Can you work these out from the model? Positions are in its coordinate system, mm. Give positions to 0.01 mm unless a question says otherwise; leave off trailing zeros. Order: outer loops, then holes, each group sorted by start corner. A loop starts at its lowest first (then second) coordinate and runs counter-clockwise, first axis right, second up. Notation, with made-up numbers: (5, 3.25) - (19, 3.25) arc R23 cw to (19, 18.25) - close; hole circle Ø10 at (19, 24.25). An arc over 180 degrees is marked (long way). Return JSON: item names as keys, results as strings.
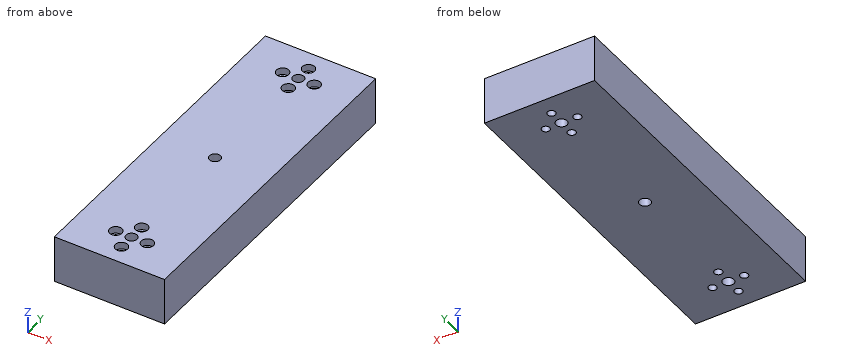
```python
from build123d import *

# Parameters (mm, degrees)
SKETCH1_W                                        = 300
SKETCH1_H                                        = 100
SKETCH1_R                                        = 5
BOSS_EXTRUDE1_DEPTH                              = 42.8
CBORE_FOR_1_4_SOCKET_HEAD_CAP_SCREW1_D           = 7.1374
CBORE_FOR_1_4_SOCKET_HEAD_CAP_SCREW1_CBORE_D     = 11.1125
CBORE_FOR_1_4_SOCKET_HEAD_CAP_SCREW1_CBORE_DEPTH = 6.35


with BuildPart() as part:
    # Sketch1 → Boss-Extrude1 (new body)
    with BuildSketch(Plane(origin=(0, 0, 0), x_dir=(0, 1, 0), z_dir=(0, 0, 1))):
        Rectangle(SKETCH1_W, SKETCH1_H)
        with Locations(Location((0, 0, 0), (0, 0, 270))):
            Circle(SKETCH1_R, mode=Mode.SUBTRACT)
        with Locations(Location((-118.5, 0, 0), (0, 0, 270))):
            Circle(SKETCH1_R, mode=Mode.SUBTRACT)
        with Locations(Location((118.5, 0, 0), (0, 0, 90))):
            Circle(SKETCH1_R, mode=Mode.SUBTRACT)
    extrude(amount=-BOSS_EXTRUDE1_DEPTH)

    # CBORE for 1/4 Socket Head Cap Screw1 (through all)
    with Locations(Plane(origin=(0, 0, 0), x_dir=(0, -1, 0), z_dir=(0, 0, 1))):
        with Locations((118.5, 14.351), (132.851, 0), (118.5, -14.351), (104.149, 0), (-104.149, 0), (-118.5, 14.351), (-132.851, 0), (-118.5, -14.351)):
            CounterBoreHole(CBORE_FOR_1_4_SOCKET_HEAD_CAP_SCREW1_D / 2, CBORE_FOR_1_4_SOCKET_HEAD_CAP_SCREW1_CBORE_D / 2, CBORE_FOR_1_4_SOCKET_HEAD_CAP_SCREW1_CBORE_DEPTH)


solid = part.part
```
1. For pin 1 Ø9.5 at (x, y) = (0, -132.851) entering from +Z; pin 2 Ø18 at (x, y) = (-14.351, 118.5) entering from -Z, each with a flat end and sliding along its axis, tell me the tip position at first contact or that it passes through.
Checks:
{"pin 1": "z = -6.35", "pin 2": "z = -42.8"}
2. Suppose I cut it at A-A (y = -118.5). List the corners of the cut face in (x, z) for me.
Checks:
{"outline": "(-50, -42.8) - (-17.92, -42.8) - (-17.92, -6.35) - (-19.91, -6.35) - (-19.91, 0) - (-50, 0) - close; (-10.78, -42.8) - (-5, -42.8) - (-5, 0) - (-8.79, 0) - (-8.79, -6.35) - (-10.78, -6.35) - close; (5, -42.8) - (10.78, -42.8) - (10.78, -6.35) - (8.79, -6.35) - (8.79, 0) - (5, 0) - close; (17.92, -42.8) - (50, -42.8) - (50, 0) - (19.91, 0) - (19.91, -6.35) - (17.92, -6.35) - close"}
3. If I drill on L1, parallel to X at y = 118, z = -14; L2, parallel to Y at x = -4, z = -14; L3, parallel to Y at x = 4.5, z = -20, over which ranges is the centre line in solid material (lowest first)? Write a range as [from, to].
Checks:
{"L1": "[-50, -17.88], [-10.82, -4.97], [4.97, 10.82], [17.88, 50]", "L2": "[-150, -121.5], [-115.5, -3], [3, 115.5], [121.5, 150]", "L3": "[-150, -120.68], [-116.32, -2.18], [2.18, 116.32], [120.68, 150]"}
4. Suppose I cut it at B-B (z = -10.5). State how many separate pieces and enclosed holes the cut face has, plus the area to 3 significant figures.
Checks:
{"separate pieces": "1", "enclosed holes": "11", "area": "29,400 mm^2"}
